```python
from build123d import *

# Parameters (mm, degrees)
F0_R     = 19.05
F0_R_2   = 8
F0_W     = 24
F0_H     = 2
F3_DEPTH = 25


# Not quite as in the source:
# - the program builds the solid bodies; features that only make, move or delete a surface that nothing else refers to are left out


with BuildPart() as f3:
    # F0 (on Front) → F3 (new body)
    with BuildSketch(Plane.XZ):
        Circle(F0_R)
        Circle(F0_R_2, mode=Mode.SUBTRACT)
        with Locations((0, 11)):
            Rectangle(F0_W, F0_H, mode=Mode.SUBTRACT)
    extrude(amount=F3_DEPTH)


solid = f3.part
```
Source: CAD feature listing. Evaluate the final solid. Frame: model axes, mm. A direction names the side the tool comes from. Round coordinates to 2 decimals unless told otherwise and drop trailing zeros. Write each loop counter-clockwise with the first axis right and the second up, starting at its lowest first coordinate (ties: lowest second). Pieces come first, ordered by that corner, then holes. Notation, with made-up numbers: M 28.5,33 L 74.5,33 A17 cw 74.5,41 Z; hole C -37.5,-29.75 d1. An arc over 180 degrees is marked long. Use CSV: the item, a comma, the result in double quotes. Start each with the question number.
Q1. Line query: line 1 (Z direction, x = 0, y = -11); line 2 (Z direction, x = 3, y = -1.5); line 3 (X direction, y = -19, z = 3). Output: solid intervals per line, ascending. Write a range as from..to.
Q2. First-contact query: P1, Ø4, axis at y = -11.5, z = -14.5, coming from the -X side; P2, Ø1.5, axis at x = -10.5, y = -6, coming from the +Z side; P3, Ø12, axis at y = -15.5, z = 13, coming from the +X side. Flat tips, straight axial feed; report the tip coordinate or a pass-through.
Q3. Cut plane C-C on y = -3.5. Output: boundary loops of the cut face in (x, z).
Q4. Access query for faces 1 (the face through (8.2, -25, 0.3)), 2 (the face through (0, -12, 10)). Directions: +Z, -Z, +X, -X, +Y, -Y. A direction counts if a zero-diameter tool reaches every point of the face in a straight line with its end or side. Return the directions, or none.
Q5. Cut plane B-B on z = 0. Output: boundary loops of the cut face in (x, y), plus the area to 4 significant figures.
Q6. Cut plane A-A on x = 0. Output: boundary loops of the cut face in (y, z).
Q7. Cut plane D-D on x = 6.5. Output: boundary loops of the cut face in (y, z), plus the area to 3 significant figures.
Q8. Pull-direction query (X, two-part tool) for faces 3 (the face through (-15.12, -12.32, -11.59)), 4 (the face through (-12, -12, 11)), 5 (the face through (8.2, 0, 0.3)); classes: +X half, -X half, draft (parallel to the pull), parting line (faces both ways), or undercut.
Results found:
1,line 1,"-19.05..-8, 8..10, 12..19.05"
1,line 2,"-18.81..-7.42, 7.42..10, 12..18.81"
1,line 3,"-18.81..-7.42, 7.42..18.81"
2,P1,"x = -14.38"
2,P2,"z = 16.37"
2,P3,"x = 17.72"
3,outline,"C 0,0 d38.1; hole M -12,10 L 12,10 L 12,12 L -12,12 Z; hole C 0,0 d16"
4,face 1,"+Z, -Z, +X, -X, -Y"
4,face 2,"+Y, -Y"
5,outline,"M -19.05,-25 L -8,-25 L -8,0 L -19.05,0 Z; M 8,-25 L 19.05,-25 L 19.05,0 L 8,0 Z"
5,area,"552.5 mm^2"
6,outline,"M -25,-19.05 L 0,-19.05 L 0,-8 L -25,-8 Z; M -25,8 L 0,8 L 0,10 L -25,10 Z; M -25,12 L 0,12 L 0,19.05 L -25,19.05 Z"
7,outline,"M -25,-17.91 L 0,-17.91 L 0,-4.66 L -25,-4.66 Z; M -25,4.66 L 0,4.66 L 0,10 L -25,10 Z; M -25,12 L 0,12 L 0,17.91 L -25,17.91 Z"
7,area,"612 mm^2"
8,face 3,"parting line"
8,face 4,"undercut"
8,face 5,"draft"
